Work out the finished part from the listing and answer in its coordinate system (mm). A direction names the side the tool comes from. Give positions to 0.01 mm unless a question says otherwise; leave off trailing zeros. Loops run counter-clockwise (first coordinate to the right, second up) from the corner with the lowest first, then second, coordinate; pieces in that order, holes last. Notation, with made-up numbers: (-21.75, 33.5) - (22.25, 33.5) arc R13 ccw to (22.25, 57.5) - close; hole circle Ø3 at (73, 86.5). An arc over 180 degrees is marked (long way). One line per question, with ' | ' between items. Start each with the question number.
1. Which of the six approach directions +Z, -Z, +X, -X, +Y, -Y give full straight-line access (tool end or side, diameter ignored) to faces 1 (the face through (12.7, 0, 2)), 2 (the face through (-6.35, 29, 2))?
2. For a pull along X with two mould halves and no side action, classify faces 3 (the face through (6.35, 28, 2)), 4 (the face through (-12.7, 0, 2)), 5 (the face through (-0.2, 0.5, 0)) as released by +X, released by -X, zero draft, split by the parting line, or undercut.
3. Section A-A (x = 0) is taken. Determine the outline of the cut face in (y, z) (3 decimals), plus the area to 3 significant figures.
4. Section B-B (y = 28.5) is taken. Determine the outline of the cut face in (x, z) (3 decimals).
5. This flat-tipped pin is pushed along its axis until it touches: pin 1 (1.5 mm diameter, centred on x = -10, y = 20.5, fed in from -Z). Where does it stop, or does it pass through?
6. Section C-C (z = 1.8) is taken. Determine the outline of the cut face in (x, y) (3 decimals).
7. Section D-D (y = 19.5) is taken. Determine the outline of the cut face in (x, z) (3 decimals).
8. Find the intervals of material crossed by line 1 (Y direction, x = 0.25, z = 1.05) (3 decimals); line 2 (Y direction, x = 0, z = 0.75) (3 decimals); line 3 (X direction, y = -3, z = 2.5), in increasing order.
from build123d import *

# Parameters (mm, degrees)
SKETCH1_W               = 25.4
SKETCH1_H               = 69.85
BOSS_EXTRUDE1_DEPTH     = 3.175
CUT_EXTRUDE1_DEPTH      = 38.297804895
F_1_4_CLEARANCE_HOLE1_D = 6.7564


with BuildPart() as part:
    # Sketch1 → Boss-Extrude1 (new body)
    with BuildSketch(Plane.XY):
        Rectangle(SKETCH1_W, SKETCH1_H)
    extrude(amount=BOSS_EXTRUDE1_DEPTH)

    # Sketch2 → Cut-Extrude1 (cut, through all)
    with BuildSketch(Plane.XY.offset(3.175)):
        with BuildLine():
            Line((-6.35, 34.925), (-6.35, 22.225))
            ThreePointArc((-6.35, 22.225), (0, 15.875), (6.35, 22.225))
            Line((6.35, 22.225), (6.35, 34.925))
            Line((6.35, 34.925), (-6.35, 34.925))
        make_face()
    extrude(amount=-CUT_EXTRUDE1_DEPTH, mode=Mode.SUBTRACT)

    # 1/4 Clearance Hole1 (through all)
    with Locations(Plane.XY.offset(3.175)):
        with Locations((0, -28.575), (0, -3.175)):
            Hole(F_1_4_CLEARANCE_HOLE1_D / 2)


solid = part.part
Conclusion:
1) face 1: +Z, -Z, +X, +Y, -Y | face 2: +Z, -Z, +Y
2) face 3: undercut | face 4: released by -X | face 5: zero draft
3) outline: (-34.925, 0) - (-31.953, 0) - (-31.953, 3.175) - (-34.925, 3.175) - close; (-25.197, 0) - (-6.553, 0) - (-6.553, 3.175) - (-25.197, 3.175) - close; (0.203, 0) - (15.875, 0) - (15.875, 3.175) - (0.203, 3.175) - close | area: 118 mm²
4) outline: (-12.7, 0) - (-6.35, 0) - (-6.35, 3.175) - (-12.7, 3.175) - close; (6.35, 0) - (12.7, 0) - (12.7, 3.175) - (6.35, 3.175) - close
5) pin 1: z = 0
6) outline: (-12.7, -34.925) - (12.7, -34.925) - (12.7, 34.925) - (6.35, 34.925) - (6.35, 22.225) arc R6.35 cw to (-6.35, 22.225) - (-6.35, 34.925) - (-12.7, 34.925) - close; hole circle Ø6.756 at (0, -28.575); hole circle Ø6.756 at (0, -3.175)
7) outline: (-12.7, 0) - (-5.736, 0) - (-5.736, 3.175) - (-12.7, 3.175) - close; (5.736, 0) - (12.7, 0) - (12.7, 3.175) - (5.736, 3.175) - close
8) line 1: -34.925 to -31.944, -25.206 to -6.544, 0.194 to 15.88 | line 2: -34.925 to -31.953, -25.197 to -6.553, 0.203 to 15.875 | line 3: -12.7 to -3.37, 3.37 to 12.7
